Verification items for this drawing (mm, ordinates from the low corner). A direction names the side the tool comes from. Round coordinates to 2 decimals unless told otherwise and drop trailing zeros. Write each loop counter-clockwise with the first axis right and the second up, starting at its lowest first coordinate (ties: lowest second). Pieces come first, ordered by that corner, then holes. Notation, with made-up numbers: (-35.75, 36) -> (-25.75, 36) arc R11 ccw to (-25.75, 44) -> close; hole circle Ø8 at (1.25, 27.25). An arc over 180 degrees is marked (long way). Use one line per item in the form item = value. Start each with the question number.
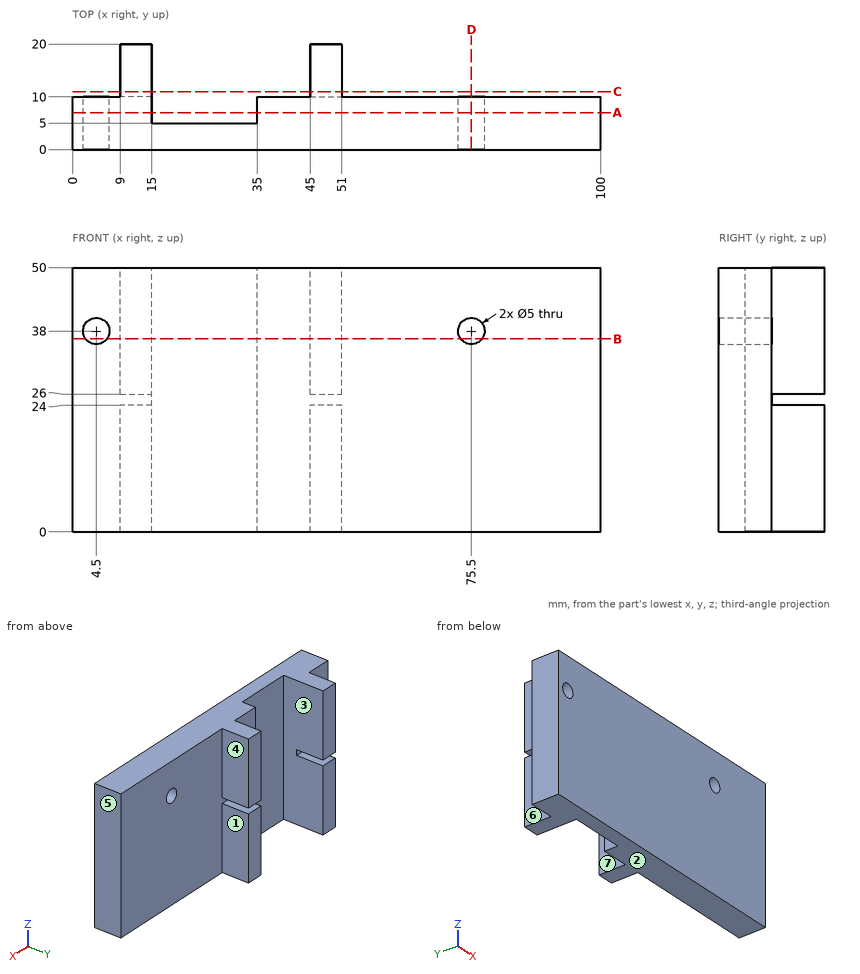
1. Tool access check on the marked faces 4, 5, 6 and 7. Record the directions out of +Z, -Z, +X, -X, +Y, -Y that give a thin tool (end or side, any length) a straight path to the whole face; none if there is none.
2. Depth check by flat-ended pin: pin 1 (4.5 mm diameter, centred on x = 4.5, z = 27, fed in from +Y); pin 2 (5 mm diameter, centred on y = 16.5, z = 11, fed in from -X); pin 3 (3 mm diameter, centred on y = 15, z = 9, fed in from +X). Enter the tip coordinate at first touch or a pass-through.
3. Sectioned sample at D-D (x = 75.5). Enter the section's corners in (y, z).
4. Sectioned sample at B-B (z = 36.5). Enter the section's corners in (x, y).
5. Sectioned sample at C-C (y = 11). Enter the section's corners in (x, z), and give its area (3 significant figures).
6. Sectioned sample at A-A (y = 7). Enter the section's corners in (x, z).
7. Mould release check, pull along X, two halves, no side actions. Record for the marked faces 1, 2 and 3: +X half, -X half, draft (parallel to the pull), parting line (faces both ways), or undercut.
8. Scan lines: probe 1 along X at (y, z) = (5.75, 38); probe 2 along X at (y, z) = (3.5, 38); probe 3 along X at (y, z) = (7.75, 20.5). Record each from-to range of solid material in increasing order.
Returned:
q1.face_4 = +Z, -Z, +X, +Y
q1.face_5 = +Z, -Z, +X, +Y, -Y
q1.face_6 = +Z, -Z, -X, +Y
q1.face_7 = +Z, -Z, +Y
q2.pin_1 = 10
q2.pin_2 = 9
q2.pin_3 = 51
q3.outline = (0, 0) -> (10, 0) -> (10, 35.5) -> (0, 35.5) -> close; (0, 40.5) -> (10, 40.5) -> (10, 50) -> (0, 50) -> close
q4.outline = (0, 0) -> (2.5, 0) -> (2.5, 10) -> (0, 10) -> close; (6.5, 0) -> (73.5, 0) -> (73.5, 10) -> (51, 10) -> (51, 20) -> (45, 20) -> (45, 10) -> (35, 10) -> (35, 5) -> (15, 5) -> (15, 20) -> (9, 20) -> (9, 10) -> (6.5, 10) -> close; (77.5, 0) -> (100, 0) -> (100, 10) -> (77.5, 10) -> close
q5.outline = (9, 0) -> (15, 0) -> (15, 24) -> (9, 24) -> close; (9, 26) -> (15, 26) -> (15, 50) -> (9, 50) -> close; (45, 0) -> (51, 0) -> (51, 24) -> (45, 24) -> close; (45, 26) -> (51, 26) -> (51, 50) -> (45, 50) -> close
q5.area = 576 mm^2
q6.outline = (0, 0) -> (15, 0) -> (15, 50) -> (0, 50) -> close; (35, 0) -> (100, 0) -> (100, 50) -> (35, 50) -> close; hole circle Ø5 at (4.5, 38); hole circle Ø5 at (75.5, 38)
q7.face_1 = +X half
q7.face_2 = draft
q7.face_3 = undercut
q8.probe_1 = 0 to 2, 7 to 15, 35 to 73, 78 to 100
q8.probe_2 = 0 to 2, 7 to 73, 78 to 100
q8.probe_3 = 0 to 15, 35 to 100
